Geometry: final body of the model. Coordinates: model frame, mm. Face numbers are marked on the shaded views. A direction names the side the tool comes from. Coordinates: 2 decimals unless noted, no trailing zeros. Loops run counter-clockwise (first coordinate to the right, second up) from the corner with the lowest first, then second, coordinate; pieces in that order, holes last. Notation, with made-up numbers: (0.25, 31) -> (12.25, 31) arc R19 cw to (12.25, 64) -> close; hole circle Ø1 at (46, 5). An arc over 180 degrees is marked (long way). One line per item, written item: value. Start each with the question number.
Item 1: Contact query for flat-ended pins moving along their axis: pin 1 Ø0.5 at (x, y) = (-5, 1.5) entering from +Z; pin 2 Ø0.6 at (x, z) = (1, -2) entering from -Y. Output: stop coordinate, or through.
Item 2: Ray query, probe 1 along Y at (x, z) = (1.25, 1.5); probe 2 along Z at (x, y) = (5, 1.5). Return the intervals inside material, ascending. Write a range as from..to.
Item 3: Section query A-A on x = -5. Return loops of the section in (y, z), then the cut area to 3 significant figures.
Item 4: Section query B-B on z = 1.55. Give the number of separate pieces and of enclosed holes in the cut face, then the cut area to 3 significant figures.
Item 5: Mould query, pull axis Y, two halves, no side actions, for the marked faces 3, 4 and 5. Classes: +Y half, -Y half, draft (parallel to the pull), parting line (faces both ways), or undercut.
Item 6: Set-up query: the marked faces 1 and 2. Return all of +Z, -Z, +X, -X, +Y, -Y with unobstructed straight access to the full face (end or side cutting, diameter ignored); none if empty.
from build123d import *

# Parameters (mm, degrees)
SKETCH1_W                  = 12.4
SKETCH1_H                  = 5.6
BOSS_EXTRUDE1_DEPTH        = 3.5
SKETCH2_W                  = 1
SKETCH2_H                  = 2.5
CUT_EXTRUDE1_DEPTH         = 4
CHAMFER1_SIZE              = 0.1
CUT_EXTRUDE2_REACH         = 10.166
SKETCH3_W                  = 0.5
SKETCH3_H                  = 0.5
CHAMFER3_SIZE              = 0.05
LPATTERN1_COUNT            = 6
LPATTERN1_PITCH            = 2
CHAMFER1_OF_LPATTERN1_SIZE = 0.1
CHAMFER3_OF_LPATTERN1_SIZE = 0.05
CHAMFER2_SIZE              = 0.1


with BuildPart() as part:
    # Sketch1 → Boss-Extrude1 (new body)
    with BuildSketch(Plane(origin=(0, 0, 0), x_dir=(1, 0, 0), z_dir=(0, 1, 0))):
        Rectangle(SKETCH1_W, SKETCH1_H)
    extrude(amount=BOSS_EXTRUDE1_DEPTH)

    # Sketch2 → Cut-Extrude1 (cut)
    with BuildSketch(Plane.XY.offset(2.8)):
        with Locations((-5, 1.75)):
            Rectangle(SKETCH2_W, SKETCH2_H)
    cut_extrude1 = extrude(amount=-CUT_EXTRUDE1_DEPTH, mode=Mode.SUBTRACT)

    # Chamfer1
    chamfer1_edges = [part.edges().sort_by_distance(p)[0] for p in [
        (-5, 3, 2.8),
        (-4.5, 1.75, 2.8),
        (-5.5, 1.75, 2.8),
        (-5, 0.5, 2.8),
    ]]
    chamfer(chamfer1_edges, length=CHAMFER1_SIZE)

    # Sketch3 → Cut-Extrude2 (cut, up to next)
    with BuildSketch(Plane.XY.offset(-1.2), mode=Mode.PRIVATE) as cut_extrude2_sk1:
        with Locations((-5, 2.25)):
            Rectangle(SKETCH3_W, SKETCH3_H)
    cut_extrude2_tool1 = extrude(cut_extrude2_sk1.sketch, amount=-CUT_EXTRUDE2_REACH, mode=Mode.PRIVATE) & part.part
    cut_extrude2 = cut_extrude2_tool1.solids().sort_by_distance((-5, 2.25, -1.2))[0]
    add(cut_extrude2, mode=Mode.SUBTRACT)

    # Chamfer3
    chamfer3_edges = [part.edges().sort_by_distance(p)[0] for p in [
        (-5.25, 2.25, -2.8),
        (-5, 2, -2.8),
        (-5, 2.5, -2.8),
        (-4.75, 2.25, -2.8),
    ]]
    chamfer(chamfer3_edges, length=CHAMFER3_SIZE)

    # LPattern1: Cut-Extrude1, Cut-Extrude2 ×6
    with Locations(*[(i * LPATTERN1_PITCH, 0, 0) for i in range(1, LPATTERN1_COUNT)]):
        add(cut_extrude1, mode=Mode.SUBTRACT)
        add(cut_extrude2, mode=Mode.SUBTRACT)

    # Chamfer1 of LPattern1
    chamfer1_of_lpattern1_edges = [part.edges().sort_by_distance(p)[0] for p in [
        (-3, 3, 2.8),
        (-2.5, 1.75, 2.8),
        (-3.5, 1.75, 2.8),
        (-3, 0.5, 2.8),
        (-1, 3, 2.8),
        (-0.5, 1.75, 2.8),
        (-1.5, 1.75, 2.8),
        (-1, 0.5, 2.8),
        (1, 3, 2.8),
        (1.5, 1.75, 2.8),
        (0.5, 1.75, 2.8),
        (1, 0.5, 2.8),
        (3, 3, 2.8),
        (3.5, 1.75, 2.8),
        (2.5, 1.75, 2.8),
        (3, 0.5, 2.8),
        (5, 3, 2.8),
        (5.5, 1.75, 2.8),
        (4.5, 1.75, 2.8),
        (5, 0.5, 2.8),
    ]]
    chamfer(chamfer1_of_lpattern1_edges, length=CHAMFER1_OF_LPATTERN1_SIZE)

    # Chamfer3 of LPattern1
    chamfer3_of_lpattern1_edges = [part.edges().sort_by_distance(p)[0] for p in [
        (-3.25, 2.25, -2.8),
        (-3, 2, -2.8),
        (-3, 2.5, -2.8),
        (-2.75, 2.25, -2.8),
        (-1.25, 2.25, -2.8),
        (-1, 2, -2.8),
        (-1, 2.5, -2.8),
        (-0.75, 2.25, -2.8),
        (0.75, 2.25, -2.8),
        (1, 2, -2.8),
        (1, 2.5, -2.8),
        (1.25, 2.25, -2.8),
        (2.75, 2.25, -2.8),
        (3, 2, -2.8),
        (3, 2.5, -2.8),
        (3.25, 2.25, -2.8),
        (4.75, 2.25, -2.8),
        (5, 2, -2.8),
        (5, 2.5, -2.8),
        (5.25, 2.25, -2.8),
    ]]
    chamfer(chamfer3_of_lpattern1_edges, length=CHAMFER3_OF_LPATTERN1_SIZE)

    # Chamfer2
    chamfer2_edges = [part.edges().sort_by_distance(p)[0] for p in [
        (6.2, 3.5, 0),
        (0, 3.5, -2.8),
        (-6.2, 3.5, 0),
        (0, 3.5, 2.8),
        (-6.2, 1.75, -2.8),
        (6.2, 1.75, -2.8),
        (6.2, 1.75, 2.8),
        (-6.2, 1.75, 2.8),
    ]]
    chamfer(chamfer2_edges, length=CHAMFER2_SIZE)


solid = part.part
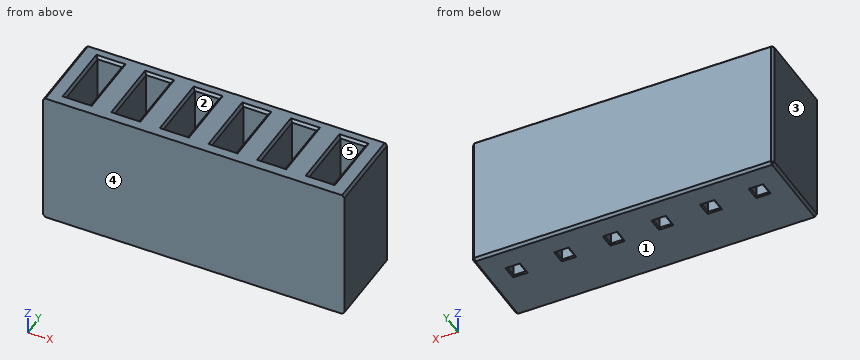
Reply:
1. pin 1: stops at z = -1.2
1. pin 2: stops at y = 0
2. probe 1: y = 0..0.5, 3..3.5
2. probe 2: z = -2.8..-1.2
3. outline: (0, -2.8) -> (1.95, -2.8) -> (2, -2.75) -> (2, -1.2) -> (0.5, -1.2) -> (0.5, 2.7) -> (0.4, 2.8) -> (0, 2.8) -> close; (2.5, -2.75) -> (2.55, -2.8) -> (3.4, -2.8) -> (3.5, -2.7) -> (3.5, 2.7) -> (3.4, 2.8) -> (3.1, 2.8) -> (3, 2.7) -> (3, -1.2) -> (2.5, -1.2) -> close
3. area: 8.78 mm²
4. separate pieces: 1
4. enclosed holes: 6
4. area: 28.4 mm²
5. face 3: draft
5. face 4: -Y half
5. face 5: undercut
6. face 1: -Z, +X, -X, +Y, -Y
6. face 2: +Z
